Geometry check sheet. Reference: the model listing, model coordinates, mm. Face numbers are marked on the shaded views. A direction names the side the tool comes from. Coordinates: 2 decimals unless noted, no trailing zeros. Order: outer loops, then holes, each group sorted by start corner. A loop starts at its lowest first (then second) coordinate and runs counter-clockwise, first axis right, second up. Notation, with made-up numbers: M 16,33 L 73,33 A24 ccw 73,70 Z; hole C -37,18.5 d10. An arc over 180 degrees is marked long. One line per item, written item: value. Start each with the question number.
1) Access from +Z, -Z, +X, -X, +Y, -Y to the whole of each face (thin tool, end or side, straight path). Record for the marked faces 1, 2 and 3.
2) Thickness scan on L1, parallel to X at y = 27, z = 0; L2, parallel to Y at x = -103, z = 41.5. Record the ranges inside material, lowest first. Write a range as from..to.
3) Go/stop test with flat-tipped pins: P1, Ø3.5, axis at x = -129, z = -5, coming from the -Y side; P2, Ø6.5, axis at x = 44.5, z = -119, coming from the -Y side; P3, Ø12.5, axis at x = 98, z = -75.5, coming from the -Y side; P4, Ø6, axis at y = 3, z = -53.5, coming from the -X side. Record where each tip stops, or that it passes through.
4) Draft check along X on the marked faces 4, 5 and 6. Enter one of: pulls with the +X half, pulls with the -X half, needs draft (parallel to the pull), parting line crosses it, or undercut.
5) Sectioned sample at B-B, the plane x = 0. Enter the section's corners in (y, z).
6) Sectioned sample at A-A, the plane y = 16. Enter the section's corners in (x, z).
```python
from build123d import *

# Parameters (mm, degrees)
STAGE1EX_DEPTH      = 30
STAGE1EX_DRAFT      = -30
STAGE1IN_DEPTH      = 27
STAGE1IN_DRAFT      = -30
SKETCH8_R           = 143.211859946
SKETCH8_R_2         = 130
BOSS_EXTRUDE2_DEPTH = 6
SKETCH15_R          = 2.38


with BuildPart() as part:
    # Sketch4 → Stage1Ex (with draft: the straight prism first)
    with BuildSketch(Plane(origin=(0, 0, 0), x_dir=(1, 0, 0), z_dir=(0, 1, 0))):
        Polygon((38.627124297, -118.882064537), (101.127124297, -73.473156537), (125, 0), (101.127124297, 73.473156537), (38.627124297, 118.882064537), (-38.627124297, 118.882064537), (-101.127124297, 73.473156537), (-125, 0), (-101.127124297, -73.473156537), (-38.627124297, -118.882064537), align=None)
    extrude(amount=STAGE1EX_DEPTH)
    # Stage1Ex: the draft: its side faces are tilted about the plane it starts from
    stage1ex_sides = [part.faces().sort_by_distance(p)[0] for p in [
        (69.877124297, 15, 96.177610537),
        (113.063562148, 15, 36.736578268),
        (113.063562148, 15, -36.736578268),
        (69.877124297, 15, -96.177610537),
        (0, 15, -118.882064537),
        (-69.877124297, 15, -96.177610537),
        (-113.063562148, 15, -36.736578268),
        (-113.063562148, 15, 36.736578268),
        (-69.877124297, 15, 96.177610537),
        (0, 15, 118.882064537),
    ]]
    draft(stage1ex_sides, Plane(origin=(0, 0, 0), x_dir=(1, 0, 0), z_dir=(0, 1, 0)), STAGE1EX_DRAFT)


with BuildPart() as stage1in_tool:
    # Sketch7 → Stage1In (with draft: the straight prism first)
    with BuildSketch(Plane(origin=(0, 30, 0), x_dir=(1, 0, 0), z_dir=(0, 1, 0))):
        Polygon((-140.223274297, 0.261449456), (-113.596688048, -82.209655607), (-43.580027974, -133.279466431), (43.082721556, -133.441051082), (113.289335779, -82.632689713), (140.223274297, -0.261449456), (113.596688048, 82.209655607), (43.580027974, 133.279466431), (-43.082721556, 133.441051082), (-113.289335779, 82.632689713), align=None)
    extrude(amount=-STAGE1IN_DEPTH)
    # Stage1In: the draft: its side faces are tilted about the plane it starts from
    stage1in_sides = [stage1in_tool.faces().sort_by_distance(p)[0] for p in [
        (-126.909981172, 16.5, 40.974103075),
        (-78.588358011, 16.5, 107.744561019),
        (-0.248653209, 16.5, 133.360258757),
        (78.186028667, 16.5, 108.036870397),
        (126.756305038, 16.5, 41.447069585),
        (126.909981172, 16.5, -40.974103075),
        (78.588358011, 16.5, -107.744561019),
        (0.248653209, 16.5, -133.360258757),
        (-78.186028667, 16.5, -108.036870397),
        (-126.756305038, 16.5, -41.447069585),
    ]]
    draft(stage1in_sides, Plane(origin=(0, 30, 0), x_dir=(1, 0, 0), z_dir=(0, 1, 0)), STAGE1IN_DRAFT)


with BuildPart() as part_1:
    add(part.part)

    # Stage1In: cut by stage1in_tool
    add(stage1in_tool.part, mode=Mode.SUBTRACT)

    # Sketch8 → Boss-Extrude2 (add)
    with BuildSketch(Plane(origin=(0, 30, 0), x_dir=(1, 0, 0), z_dir=(0, 1, 0))):
        with Locations(Location((0, 0, 0), (0, 0, 270))):
            Circle(SKETCH8_R)
        with Locations(Location((0, 0, 0), (0, 0, 270))):
            Circle(SKETCH8_R_2, mode=Mode.SUBTRACT)
    extrude(amount=-BOSS_EXTRUDE2_DEPTH)

    # Cut-Sweep1: sweep along a path in Sketch14
    with BuildLine(Plane(origin=(0, 30, 0), x_dir=(1, 0, 0), z_dir=(0, 1, 0))) as cut_sweep1_path:
        CenterArc((0, 0), 136, 0, 360)
    # Sketch15 → Cut-Sweep1 (sweep, cut)
    with BuildSketch(Plane(origin=(0, 0, 0), x_dir=(-0.9999982617823745, 0, -0.0018645193026112638), z_dir=(0.0018645193026112638, 0, -0.9999982617823745))):
        with Locations((-135.972501612, 31.5)):
            Circle(SKETCH15_R)
    sweep(path=cut_sweep1_path.line, mode=Mode.SUBTRACT)


solid = part_1.part
```
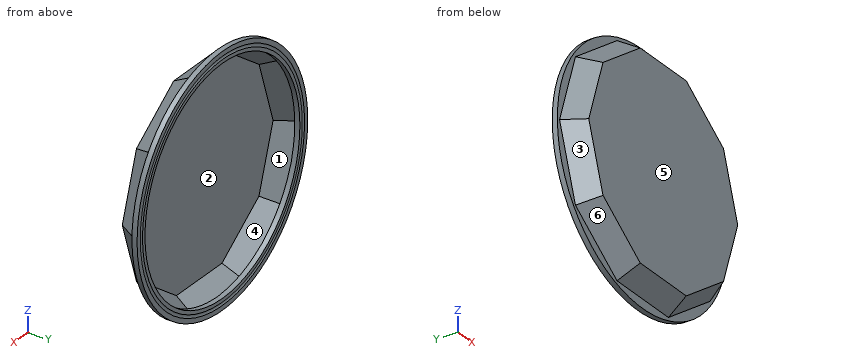
Final values:
1. face 1: none
1. face 2: +Y
1. face 3: -Z, -X, -Y
2. L1: x = -143.21..-130, 130..143.21
2. L2: y = 0..3
3. P1: stops at y = 6.23
3. P2: stops at y = 0.52
3. P3: stops at y = 0
3. P4: stops at x = -111.5
4. face 4: undercut
4. face 5: needs draft
4. face 6: pulls with the -X half
5. outline: M 0,-118.88 L 24,-132.74 L 24,-143.21 L 30,-143.21 L 30,-137.82 A2.38 cw 30,-134.12 L 30,-130 L 24.18,-130 L 3,-117.77 L 3,117.77 L 24.18,130 L 30,130 L 30,134.12 A2.38 cw 30,137.82 L 30,143.21 L 24,143.21 L 24,132.74 L 0,118.88 Z
6. outline: M -134.71,0 L -108.99,-79.18 L -41.63,-128.12 L 41.63,-128.12 L 108.99,-79.18 L 134.71,0 L 108.99,79.18 L 41.63,128.12 L -41.63,128.12 L -108.99,79.18 Z; hole M -131.72,-0.25 L -106.42,-77.62 L -40.47,-125.35 L 40.94,-125.2 L 106.71,-77.23 L 131.72,0.25 L 106.42,77.62 L 40.47,125.35 L -40.94,125.2 L -106.71,77.23 Z
